```python
from build123d import *

# Parameters (mm, degrees)
F0_W     = 18
F0_H     = 26
F1_DEPTH = 1.6
F2_R     = 2.9
F3_DEPTH = 4.4
F4_W     = 4.789572
F4_H     = 3.672005
F4_W_2   = 2.95357
F4_H_2   = 4.550093
F5_DEPTH = 1.5
F6_R     = 0.75
F6_R_2   = 0.5
F7_DEPTH = 25


with BuildPart() as f1:
    # F0 (on Top) → F1 (new body)
    with BuildSketch(Plane.XY):
        Rectangle(F0_W, F0_H)
    extrude(amount=F1_DEPTH)

    # F2 (on face) → F3 (join)
    with BuildSketch(Plane.XY.offset(1.6)):
        with Locations((3, 7)):
            Circle(F2_R)
    extrude(amount=F3_DEPTH)

    # F4 (on face) → F5 (join)
    with BuildSketch(Plane.XY.offset(1.6)):
        with Locations((-5.280366, 5.431945)):
            Rectangle(F4_W, F4_H)
        with Locations((-0.131576, -0.03615)):
            Rectangle(F4_W_2, F4_H_2)
    extrude(amount=F5_DEPTH)

    # F6 (on face) → F7 (cut)
    with BuildSketch(Plane.XY.offset(1.6)):
        with Locations((-2.5, -11.5)):
            Circle(F6_R)
        with Locations((2.5, -11.5)):
            Circle(F6_R)
        with Locations((7.5, 11.5)):
            Circle(F6_R_2)
        with Locations((-7.5, 11.5)):
            Circle(F6_R_2)
    extrude(amount=-F7_DEPTH, mode=Mode.SUBTRACT)


solid = f1.part
```
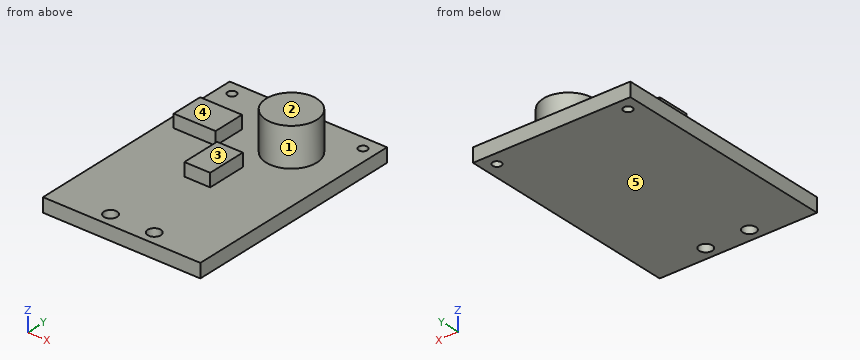
Can you work these out from the model? Positions are in its coordinate system, mm. Face numbers are marked on the shaded views. A direction names the side the tool comes from. Coordinates: 2 decimals unless noted, no trailing zeros. Loops run counter-clockwise (first coordinate to the right, second up) from the corner with the lowest first, then second, coordinate; pieces in that order, holes last.
1) Imagine slicing it at D-D on y = 0.5. List the corners of the cut face in (x, z) for me, plus the area to 3 significant figures.
2) For pin 1 (2.5 mm diameter, centred on x = 0, y = -0.5, fed in from +Z); pin 2 (5 mm diameter, centred on x = 4.5, y = -5.5, fed in from +Z); pin 3 (0.8 mm diameter, centred on y = 6, z = 2.5, fed in from +X), each with a flat end and sliding along its axis, tell me the tip position at first contact or that it passes through.
3) Imagine slicing it at C-C on x = 7.5. List the corners of the cut face in (y, z) for me.
4) Imagine slicing it at A-A on z = 2.35. List the corners of the cut face in (x, y) for me, plus the area to 3 significant figures.
5) Which directions (+Z, -Z, +X, -X, +Y, -Y) give clear straight access to the entire face, cutting with the end or side of a thin tool? Please do the marked faces 1, 2, 3, 4 and 5.
6) Imagine slicing it at B-B on y = 11.5. List the corners of the cut face in (x, z) for me.
7) I need wall thicknesses on probe 1 along Y at (x, z) = (7.5, 0.6); probe 2 along Y at (x, z) = (2.5, 0.65); probe 3 along Z at (x, y) = (-1.5, 11). Which ranges of each line are inside material? Lowest first, please.
Completed:
1. outline: (-9, 0) - (9, 0) - (9, 1.6) - (1.35, 1.6) - (1.35, 3.1) - (-1.61, 3.1) - (-1.61, 1.6) - (-9, 1.6) - close
1. area: 33.2 mm2
2. pin 1: stops at z = 3.1
2. pin 2: stops at z = 1.6
2. pin 3: stops at x = 5.84
3. outline: (-13, 0) - (11, 0) - (11, 1.6) - (-13, 1.6) - close; (12, 0) - (13, 0) - (13, 1.6) - (12, 1.6) - close
4. outline: (-7.68, 3.6) - (-2.89, 3.6) - (-2.89, 7.27) - (-7.68, 7.27) - close; (-1.61, -2.31) - (1.35, -2.31) - (1.35, 2.24) - (-1.61, 2.24) - close; circle Ø5.8 at (3, 7)
4. area: 57.4 mm2
5. face 1: +Z
5. face 2: +Z, +X, -X, +Y, -Y
5. face 3: +Z, +X, -X, -Y
5. face 4: +Z, -X, +Y, -Y
5. face 5: -Z, +X, -X, +Y, -Y
6. outline: (-9, 0) - (-8, 0) - (-8, 1.6) - (-9, 1.6) - close; (-7, 0) - (7, 0) - (7, 1.6) - (-7, 1.6) - close; (8, 0) - (9, 0) - (9, 1.6) - (8, 1.6) - close
7. probe 1: y = -13 to 11, 12 to 13
7. probe 2: y = -13 to -12.25, -10.75 to 13
7. probe 3: z = 0 to 1.6
